For this review, take the finished solid that the model builds, in its own axes (mm). A direction names the side the tool comes from. Give positions to 0.01 mm unless a question says otherwise; leave off trailing zeros. Loops run counter-clockwise (first coordinate to the right, second up) from the corner with the lowest first, then second, coordinate; pieces in that order, holes last. Notation, with made-up numbers: M -3,8.25 L 39,8.25 A17 cw 39,18.25 Z; hole C 72,55.5 d5. An arc over 180 degrees is marked long. Use CSV: the item, a comma, the result in double quotes. Start each with the question number.
1. Tool access review of faces 1 (the face through (58, 59, 4)), 2 (the face through (71, 7, 8)), 3 (the face through (15, 59, 3)): name each direction out of +Z, -Z, +X, -X, +Y, -Y from which nothing blocks a thin tool from reaching the whole face with its end or side.
2. Take a section at A-A, the plane z = 10. State how many separate pieces and enclosed holes the cut face has, and give its area (3 significant figures).
3. Take a section at D-D, the plane z = 5.5. Write out the cut boundary in (x, y).
4. Insertion check: P1, Ø5, axis at x = 71, y = 54.5, coming from the +Z side; P2, Ø0.6, axis at y = 59.5, z = 10, coming from the -X side; P3, Ø1.3, axis at x = 6.5, y = 53, coming from the +Z side; P4, Ø3, axis at x = 62, y = 42, coming from the +Z side. Each pin has a flat end and moves straight along its axis. Give the tip position at first contact, or say it passes through.
5. To check wall thickness, follow line 1 (Y direction, x = 6.5, z = 13.5); line 2 (Y direction, x = 46, z = 14.5); line 3 (X direction, y = 5, z = 7.75). State the ranges of each line that lie inside material, in increasing order. Write a range as [from, to].
6. The part is to be moulded in two halves that separate along X. For faces 4 (the face through (0, 30, 10)), 5 (the face through (40, 30, 2)), 6 (the face through (77.01, 29.46, 7.56)), say which applies: pulls with the +X half, pulls with the -X half, needs draft (parallel to the pull), parting line crosses it, or undercut.
7. Take a section at B-B, the plane y = 53.5. Write out the cut boundary in (x, z).
8. Take a section at C-C, the plane x = 47.5. Write out the cut boundary in (y, z), and give its area (3 significant figures).
from build123d import *

# Parameters (mm, degrees)
SKETCH_W        = 78
SKETCH_H        = 60
PAD_DEPTH       = 20
POCKET_DEPTH    = 18
SKETCH002_W     = 74
SKETCH002_H     = 56
POCKET001_DEPTH = 2
SKETCH003_R     = 2.25
POCKET002_DEPTH = 10
SKETCH004_R     = 2.5
POCKET003_DEPTH = 2
SKETCH005_R     = 2.5
POCKET004_DEPTH = 2
SKETCH006_W     = 5
SKETCH006_H     = 2
POCKET005_DEPTH = 60.001


with BuildPart() as part:
    # Sketch → Pad (new body)
    with BuildSketch(Plane.XY):
        with Locations((39, 30)):
            Rectangle(SKETCH_W, SKETCH_H)
    extrude(amount=PAD_DEPTH)

    # Sketch001 (on Face6 of Pad) → Pocket (cut)
    with BuildSketch(Plane.XY.offset(20)):
        Polygon((2, 50), (2, 10), (10, 10), (10, 2), (68, 2), (68, 10), (76, 10), (76, 50), (68, 50), (68, 58), (10, 58), (10, 50), align=None)
    extrude(amount=-POCKET_DEPTH, mode=Mode.SUBTRACT)

    # Sketch002 (on Face5 of Pocket) → Pocket001 (cut)
    with BuildSketch(Plane.XY.offset(20)):
        with Locations((39, 30)):
            Rectangle(SKETCH002_W, SKETCH002_H)
    extrude(amount=-POCKET001_DEPTH, mode=Mode.SUBTRACT)

    # Sketch003 (on Face26 of Pocket001) → Pocket002 (cut)
    with BuildSketch(Plane.XY.offset(18)):
        with Locations((6.5, 53.5)):
            Circle(SKETCH003_R)
        with Locations((71.5, 53.5)):
            Circle(SKETCH003_R)
        with Locations((6.5, 6.5)):
            Circle(SKETCH003_R)
        with Locations((71.5, 6.5)):
            Circle(SKETCH003_R)
    extrude(amount=-POCKET002_DEPTH, mode=Mode.SUBTRACT)

    # Sketch004 (on Face3 of Pocket002) → Pocket003 (cut)
    with BuildSketch(Plane.YZ.offset(78)):
        with Locations((30, 10)):
            Circle(SKETCH004_R)
    extrude(amount=-POCKET003_DEPTH, mode=Mode.SUBTRACT)

    # Sketch005 (on Face6 of Pocket003) → Pocket004 (cut)
    with BuildSketch(Plane(origin=(0, 60, 0), x_dir=(-1, 0, 0), z_dir=(0, 1, 0))):
        with Locations((-25, 10)):
            Circle(SKETCH005_R)
        with BuildLine():
            Line((-63.5, 7.602084), (-63.5, 12.397916))
            ThreePointArc((-52.5, 12.397916), (-58, 16), (-63.5, 12.397916))
            Line((-52.5, 7.602084), (-52.5, 12.397916))
            ThreePointArc((-63.5, 7.602084), (-58, 4), (-52.5, 7.602084))
        make_face()
    extrude(amount=-POCKET004_DEPTH, mode=Mode.SUBTRACT)

    # Sketch006 (on Face6 of Pocket004) → Pocket005 (cut, through all)
    with BuildSketch(Plane(origin=(0, 60, 0), x_dir=(-1, 0, 0), z_dir=(0, 1, 0))):
        with Locations((-65.5, 3)):
            Rectangle(SKETCH006_W, SKETCH006_H)
        with Locations((-12.5, 3)):
            Rectangle(SKETCH006_W, SKETCH006_H)
    extrude(amount=-POCKET005_DEPTH, mode=Mode.SUBTRACT)


solid = part.part
Result set:
1,face 1,"+Y"
1,face 2,"+Z"
1,face 3,"+Y, -Y"
2,separate pieces,"3"
2,enclosed holes,"4"
2,area,"686 mm2"
3,outline,"M 0,0 L 78,0 L 78,60 L 61.97,60 L 61.97,58 L 68,58 L 68,50 L 76,50 L 76,10 L 68,10 L 68,2 L 10,2 L 10,10 L 2,10 L 2,50 L 10,50 L 10,58 L 54.03,58 L 54.03,60 L 0,60 Z"
4,P1,"z = 18"
4,P2,"x = 0"
4,P3,"z = 8"
4,P4,"z = 2"
5,line 1,"[0, 4.25], [8.75, 10], [50, 51.25], [55.75, 60]"
5,line 2,"[0, 2], [58, 60]"
5,line 3,"[0, 10], [68, 78]"
6,face 4,"pulls with the -X half"
6,face 5,"undercut"
6,face 6,"needs draft"
7,outline,"M 0,0 L 78,0 L 78,20 L 76,20 L 76,18 L 73.75,18 L 73.75,8 L 69.25,8 L 69.25,18 L 68,18 L 68,2 L 10,2 L 10,18 L 8.75,18 L 8.75,8 L 4.25,8 L 4.25,18 L 2,18 L 2,20 L 0,20 Z"
8,outline,"M 0,0 L 60,0 L 60,20 L 58,20 L 58,2 L 2,2 L 2,20 L 0,20 Z"
8,area,"192 mm2"
